from build123d import *

# Parameters (mm, degrees)
SKETCH1_W           = 25
SKETCH1_H           = 22
BOSS_EXTRUDE1_DEPTH = 60
CUT_EXTRUDE2_REACH  = 123.15
CUT_EXTRUDE3_REACH  = 123.15
SKETCH6_R           = 6.26
FILLET1_R           = 5
SKETCH2_R           = 3
BOSS_EXTRUDE2_DEPTH = 10
LPATTERN1_COUNT     = 6
LPATTERN1_PITCH     = 20
SKETCH3_R           = 3
BOSS_EXTRUDE3_DEPTH = 10
LPATTERN2_COUNT     = 6
LPATTERN2_PITCH     = 20
SKETCH4_R           = 8
SKETCH4_W           = 3
SKETCH4_H           = 11
CUT_EXTRUDE1_DEPTH  = 15


with BuildPart() as part:
    # Sketch1 → Boss-Extrude1 (new, symmetric)
    with BuildSketch(Plane(origin=(0, 0, 0), x_dir=(0, 0, -1), z_dir=(1, 0, 0))):
        Rectangle(SKETCH1_W, SKETCH1_H)
    extrude(amount=BOSS_EXTRUDE1_DEPTH, both=True)

    # Sketch5 → Cut-Extrude2 (cut, up to next)
    with BuildSketch(Plane(origin=(60, 0, 0), x_dir=(0, 0, -1), z_dir=(1, 0, 0)), mode=Mode.PRIVATE) as cut_extrude2_sk1:
        with BuildLine():
            Line((-13.743342576, 11), (-11.25, 11))
            Line((-11.25, 11), (-11.25, 6.005))
            ThreePointArc((-11.25, 6.005), (-23.092030441, 3.213639122), (-13.743342576, 11))
        make_face()
    cut_extrude2_tool1 = extrude(cut_extrude2_sk1.sketch, amount=-CUT_EXTRUDE2_REACH, mode=Mode.PRIVATE) & part.part
    add(cut_extrude2_tool1.solids().sort_by_distance((60, 6.117758, 17.335764))[0], mode=Mode.SUBTRACT)

    # Sketch6 → Cut-Extrude3 (cut, up to next)
    with BuildSketch(Plane.ZY.offset(60), mode=Mode.PRIVATE) as cut_extrude3_sk1:
        with Locations((17.5, -6.005)):
            Circle(SKETCH6_R)
    cut_extrude3_tool1 = extrude(cut_extrude3_sk1.sketch, amount=-CUT_EXTRUDE3_REACH, mode=Mode.PRIVATE) & part.part
    add(cut_extrude3_tool1.solids().sort_by_distance((-60, -6.005, 17.5))[0], mode=Mode.SUBTRACT)

    # Fillet1
    fillet1_edges = [part.edges().sort_by_distance(p)[0] for p in [
        (0, 11, 11.25),
    ]]
    fillet(fillet1_edges, radius=FILLET1_R)

    # Sketch2 → Boss-Extrude2 (add)
    with BuildSketch(Plane(origin=(60, 0, 0), x_dir=(0, 0, -1), z_dir=(1, 0, 0))):
        with BuildLine():
            Line((-17.250000617, 1.202041029), (-6.000000617, 1.202041029))
            Line((-6.000000617, 1.202041029), (-6.000000617, 11))
            Line((-6.000000617, 11), (-17.250000617, 11))
            ThreePointArc((-17.250000617, 11), (-21.250000617, 6.101020514), (-17.250000617, 1.202041029))
        make_face()
        with Locations((-16.250000617, 6.101020514)):
            Circle(SKETCH2_R, mode=Mode.SUBTRACT)
    boss_extrude2 = extrude(amount=-BOSS_EXTRUDE2_DEPTH)

    # LPattern1: Boss-Extrude2 ×6
    with Locations(*[(-i * LPATTERN1_PITCH, 0, 0) for i in range(1, LPATTERN1_COUNT)]):
        add(boss_extrude2)

    # Sketch3 → Boss-Extrude3 (add)
    with BuildSketch(Plane.ZY.offset(60)):
        with BuildLine():
            Line((17.24, -1.202041029), (12.5, -1.202041029))
            Line((12.5, -1.202041029), (12.5, -2.238356932))
            ThreePointArc((12.5, -2.238356932), (11.24, -6.005), (12.5, -9.771643068))
            Line((12.5, -9.771643068), (12.5, -11))
            Line((12.5, -11), (17.24, -11))
            ThreePointArc((17.24, -11), (21.24, -6.101020514), (17.24, -1.202041029))
        make_face()
        with Locations((16.24, -6.101020514)):
            Circle(SKETCH3_R, mode=Mode.SUBTRACT)
    boss_extrude3 = extrude(amount=-BOSS_EXTRUDE3_DEPTH)

    # LPattern2: Boss-Extrude3 ×6
    with Locations(*[(i * LPATTERN2_PITCH, 0, 0) for i in range(1, LPATTERN2_COUNT)]):
        add(boss_extrude3)

    # Sketch4 → Cut-Extrude1 (cut)
    with BuildSketch(Plane(origin=(0, 0, -12.5), x_dir=(-1, 0, 0), z_dir=(0, 0, -1))):
        with Locations(Location((0, 0, 0), (0, 0, 90))):
            Circle(SKETCH4_R)
        with Locations((-14, 0)):
            Rectangle(SKETCH4_W, SKETCH4_H)
        with Locations((14, 0)):
            Rectangle(SKETCH4_W, SKETCH4_H)
    extrude(amount=-CUT_EXTRUDE1_DEPTH, mode=Mode.SUBTRACT)


solid = part.part
Here's how the part is built. I have some questions about the finished solid (model axes, mm). A direction names the side the tool comes from. Coordinates: 2 decimals unless noted, no trailing zeros. Write each loop counter-clockwise with the first axis right and the second up, starting at its lowest first coordinate (ties: lowest second). Pieces come first, ordered by that corner, then holes.
Item 1: Will these pins go through, and if not, where does the flat tip stop? pin 1 (9.5 mm diameter, centred on y = 6.1, z = 16.25, fed in from -X); pin 2 (2.5 mm diameter, centred on x = -57, z = 16, fed in from +Y); pin 3 (1.5 mm diameter, centred on x = -10.5, y = 7.5, fed in from +Z).
Item 2: If we mould it in two halves opening along Y, with no side actions, what happens to faces 1 (the flat face through (-14, -5.5, -5)), 2 (the cylindrical face through (-5.07, -5.95, 11.24)), 3 (the flat face through (-15, -1.202, 15)), 4 (the flat face through (1, 0, 12.5))? For each: +Y half, -Y half, draft (parallel to the pull), parting line (faces both ways), or undercut.
Item 3: If I drill on line 1 (X direction, y = -5, z = 20); line 2 (X direction, y = 0, z = -1.75); line 3 (Y direction, x = -13, z = 16), over which ranges is the centre line in solid material (lowest first)?
Item 4: I want a section at C-C on x = 14. Write out the boundary of the cut face in (y, z) (3 decimals).
Item 5: I want a section at D-D on x = -24. Write out the boundary of the cut face in (y, z) (3 decimals).
Item 6: I want a section at B-B on z = -5. Write out the boundary of the cut face in (x, y).
Item 7: I want a section at A-A on y = 0. Write out the boundary of the cut face in (x, z), and give its area (3 significant figures).
Item 8: On a 3-axis mill with a long thin cutter (end or side, diameter ignored), from which of +Z, -Z, +X, -X, +Y, -Y can I reach the whole of each face in a straight line? I mean faces 5 (the flat face through (45, -1.202, 15)), 6 (the cylindrical face through (54.93, -5.95, 11.24)), 7 (the flat face through (14, -5.5, -5)), 8 (the flat face through (0, 8.3, 13.9)), 9 (the flat face through (15, 1.202, 15)). Say none if no direction works.
Findings below:
1. pin 1: stops at x = -50
1. pin 2: stops at y = -1.2
1. pin 3: stops at z = 21.18
2. face 1: undercut
2. face 2: undercut
2. face 3: +Y half
2. face 4: draft
3. line 1: x = -60 to -50, -40 to -30, -20 to -10, 0 to 10, 20 to 30, 40 to 50
3. line 2: x = -60 to -15.5, -12.5 to -8, 8 to 12.5, 15.5 to 60
3. line 3: y = -11 to -9.09, -3.11 to -1.2
4. outline: (-11, -12.5) - (-5.5, -12.5) - (-5.5, 2.5) - (5.5, 2.5) - (5.5, -12.5) - (11, -12.5) - (11, 17.25) arc R5 ccw to (1.202, 17.25) - (1.202, 12.5) - (-2.238, 12.5) arc R6.26 cw to (-9.772, 12.5) - (-11, 12.5) - close; hole circle Ø6 at (6.101, 16.25)
5. outline: (-11, -12.5) - (11, -12.5) - (11, 17.25) arc R5 ccw to (1.202, 17.25) - (1.202, 12.5) - (-2.238, 12.5) arc R6.26 cw to (-9.772, 12.5) - (-11, 12.5) - close; hole circle Ø6 at (6.101, 16.25)
6. outline: (-60, -11) - (60, -11) - (60, 11) - (-60, 11) - close; hole (-15.5, -5.5) - (-12.5, -5.5) - (-12.5, 5.5) - (-15.5, 5.5) - close; hole circle Ø16 at (0, 0); hole (12.5, -5.5) - (15.5, -5.5) - (15.5, 5.5) - (12.5, 5.5) - close
7. outline: (-60, -12.5) - (-15.5, -12.5) - (-15.5, 2.5) - (-12.5, 2.5) - (-12.5, -12.5) - (-8, -12.5) - (-8, 2.5) - (8, 2.5) - (8, -12.5) - (12.5, -12.5) - (12.5, 2.5) - (15.5, 2.5) - (15.5, -12.5) - (60, -12.5) - (60, 12.5) - (-60, 12.5) - close
7. area: 2,670 mm2
8. face 5: +Z, +X, -X, +Y
8. face 6: +Z, +X
8. face 7: -Z
8. face 8: +Z, +Y
8. face 9: +Z, +X, -X, -Y
